Autodesk Inventor part; units mm, degrees
ref_plane "YZ Plane" through (0, 0, 0) normal (1, 0, 0) x (0, 1, 0)
ref_plane "XZ Plane" through (0, 0, 0) normal (0, 1, 0) x (-1, 0, 0)
ref_plane "XY Plane" through (0, 0, 0) normal (0, 0, 1) x (1, 0, 0)
sketch "Sketch1" plane through (0, 0, 0) normal (1, 0, 0) x (0, 1, 0)
  line L0 (0, 0) -> (3, 0)
  line L1 (3, 0) -> (3, -8.5)
  line L2 (3, -25.7) -> (3, -34.2)
  line L3 (3, -34.2) -> (0, -34.2)
  line L4 (0, -34.2) -> (0, -25.7)
  line L5 (0, -25.7) -> (0, -23.2)
  line L6 (0, -23.2) -> (13.7, -23.2)
  line L7 (0, 0) -> (0, -8.5)
  line L8 (0, -8.5) -> (0, -11)
  line L9 (0, -11) -> (13.7, -11)
  line L10 (13.7, -11) -> (13.7, -23.2)
  line L11 (3, -8.5) -> (3, -9)
  line L12 (3, -25.7) -> (3, -25.2)
  line L13 (3, -9) -> (15.95, -9)
  line L14 (3, -25.2) -> (15.95, -25.2)
  line L15 (15.95, -25.2) -> (15.95, -9)
  dimension "d0" = 3
  dimension "d1" = 8.5
  dimension "d4" = 8.5
  dimension "d8" = 3
  dimension "d12" = 13.7
  dimension "d14" = 12.2
  dimension "d28" = 0.5
  dimension "d29" = 0.5
  dimension "d30" = 2.25
extrude "Extrusion1" add sketch "Sketch1" against normal blind 8
sketch "Sketch3" plane through (0, 3, 0) normal (0, 1, 0) x (1, 0, 0)
  circle A0 centre (-4, 29.8) radius 2.25
  line L0 (0, 34.2) -> (-8, 34.2)
  line L1 (0, 34.2) -> (0, 25.2)
  line L2 (0, 0) -> (-8, 0)
  line L3 (0, 9) -> (0, 0)
  circle A1 centre (-4, 4.4) radius 2.25
  point P0 (0, 25.8)
  point P1 (0, 8.5)
  dimension "d16" = 4.5
  dimension "d18" = 4.4
  dimension "d19" = 4
  dimension "d23" = 4.5
  dimension "d24" = 4
  dimension "d25" = 4.4
extrude "Extrusion2" cut sketch "Sketch3" against normal through all
fillet "Fillet1" radius 2 2 edges at (-4, 15.95, -9) (-4, 15.95, -25.2)
properties part number "Linear Actuator Mount"
Can you work these out from the model? Positions are in its coordinate system, mm. A direction names the side the tool comes from. Round coordinates to 2 decimals unless told otherwise and drop trailing zeros. Loops run counter-clockwise (first coordinate to the right, second up) from the corner with the lowest first, then second, coordinate; pieces in that order, holes last.
Item 1: Will these pins go through, and if not, where does the flat tip stop? pin 1 Ø4 at (x, z) = (-2.5, -19.5) entering from -Y; pin 2 Ø4 at (x, y) = (-3.5, 7.5) entering from +Z.
Item 2: Please list where these lines run through material, in increasing order: L1, parallel to Z at x = -4, y = 1.45; L2, parallel to Z at x = -2.5, y = 8.5; L3, parallel to X at y = 1.85, z = -4.4.
Item 3: Suppose I cut it at A-A, the plane x = -4. Write out the boundary of the cut face in (y, z).
Item 4: Suppose I cut it at C-C, the plane y = 4. Write out the boundary of the cut face in (x, z).
Item 5: Suppose I cut it at B-B, the plane z = -4.4. Write out the boundary of the cut face in (x, y), then the cut area to 3 significant figures.
Item 6: Which directions (+Z, -Z, +X, -X, +Y, -Y) give clear straight access to the entire face, cutting with the end or side of a thin tool? Please do faces 1 (the flat face through (-7, 3, -4)), 2 (the flat face through (-4, 7, -23.2)), 3 (the flat face through (-8, 6.2, -23.4)), 4 (the flat face through (-4, 8, -25.2)).
Item 7: Suppose I cut it at D-D, the plane x = -6.75. Write out the boundary of the cut face in (y, z), then the cut area to 3 significant figures.
Item 8: If we mould it in two halves opening along X, with no side actions, what happens to faces 5 (the cylindrical face through (-2.962, 1.521, -27.804)), 6 (the flat face through (0, 6.2, -23.4)), 7 (the flat face through (-7, 3, -30))? For each: +X half, -X half, draft (parallel to the pull), parting line (faces both ways), or undercut.
Reported:
1. pin 1: stops at y = 13.7
1. pin 2: stops at z = -9
2. L1: z = -34.2 to -32.05, -27.55 to -23.2, -11 to -6.65, -2.15 to 0
2. L2: z = -25.2 to -23.2, -11 to -9
2. L3: x = -8 to -6.25, -1.75 to 0
3. outline: (0, -34.2) - (3, -34.2) - (3, -32.05) - (0, -32.05) - close; (0, -27.55) - (3, -27.55) - (3, -25.2) - (13.95, -25.2) arc R2 ccw to (15.95, -23.2) - (15.95, -11) arc R2 ccw to (13.95, -9) - (3, -9) - (3, -6.65) - (0, -6.65) - (0, -11) - (13.7, -11) - (13.7, -23.2) - (0, -23.2) - close; (0, -2.15) - (3, -2.15) - (3, 0) - (0, 0) - close
4. outline: (-8, -25.2) - (0, -25.2) - (0, -23.2) - (-8, -23.2) - close; (-8, -11) - (0, -11) - (0, -9) - (-8, -9) - close
5. outline: (-8, 0) - (-6.25, 0) - (-6.25, 3) - (-8, 3) - close; (-1.75, 0) - (0, 0) - (0, 3) - (-1.75, 3) - close
5. area: 10.5 mm2
6. face 1: +Z, +X, -X, +Y
6. face 2: +X, -X, -Y
6. face 3: +Z, -Z, -X, +Y, -Y
6. face 4: -Z, +X, -X, +Y
7. outline: (0, -34.2) - (3, -34.2) - (3, -25.2) - (13.95, -25.2) arc R2 ccw to (15.95, -23.2) - (15.95, -11) arc R2 ccw to (13.95, -9) - (3, -9) - (3, 0) - (0, 0) - (0, -11) - (13.7, -11) - (13.7, -23.2) - (0, -23.2) - close
7. area: 144 mm2
8. face 5: undercut
8. face 6: +X half
8. face 7: draft
